Check sheet for the modelled part. Datum: model origin and axes. Units: mm. A direction names the side the tool comes from. Coordinates: 2 decimals unless noted, no trailing zeros. Write each loop counter-clockwise with the first axis right and the second up, starting at its lowest first coordinate (ties: lowest second). Pieces come first, ordered by that corner, then holes. Notation, with made-up numbers: (47, 85.5) - (53, 85.5) arc R20 cw to (53, 112.5) - close; hole circle Ø6 at (26.5, 0.5). An arc over 180 degrees is marked (long way). Use one line per item in the form item = value. Start each with the question number.
1. Draft check along Y on faces 1 (the face through (-1.5, 0.75, 0)), 2 (the face through (0, 1, -1)), 3 (the face through (-0.91, -1.9, -0.08)), 4 (the face through (-1.5, -0.75, 0)). Enter one of: +Y half, -Y half, draft (parallel to the pull), parting line (faces both ways), or undercut.
2. Scan lines: line 1 along X through (y, z) = (1.35, -0.55); line 2 along Y through (x, z) = (6.25, 0.9). Record each from-to range of solid material in increasing order.
3. Go/stop test with a flat-tipped pin: pin 1 Ø1.5 at (x, z) = (4, 1.5) entering from -Y. Record where the tip stops, or that it passes through.
4. Tool access check on faces 5 (the face through (-0.53, 0.05, -0.02)), 6 (the face through (8, 0, 1)). Record the directions out of +Z, -Z, +X, -X, +Y, -Y that give a thin tool (end or side, any length) a straight path to the whole face; none if there is none.
5. Cross-section at A-A on x = 12.5. Record the boundary of the cut face in (y, z), then the cut area to 3 significant figures.
Autodesk Inventor part; units mm, degrees
ref_plane "Work Plane1" through (29, 0, 0) normal (0, -1, 0) x (1, 0, 0)
ref_plane "YZ Plane" through (0, 0, 0) normal (1, 0, 0) x (0, 1, 0)
ref_plane "XZ Plane" through (0, 0, 0) normal (0, 1, 0) x (-1, 0, 0)
sketch "Sketch1" plane through (0, 0, 0) normal (0, 0, 1) x (1, 0, 0)
  line L0 (-0.5, 0) -> (16, 0)
  line L1 (16, 0) -> (16, 1)
  line L2 (16, 1) -> (1, 1)
  line L3 (1, 1) -> (0.7545, 1)
  line L4 (0.7545, 1) -> (0, 1)
  line L5 (0, 1) -> (0, 1.9)
  line L6 (0, 1.9) -> (-2, 1.9)
  line L7 (-2, 1.9) -> (-2, 0.866)
  line L8 (-2, 0.866) -> (-1, 0.866)
  line L9 (-1, 0.866) -> (-0.5, 0)
  line L10 (-5.6, 0) -> (19.6, 0)
  line L11 (0, -0.38) -> (0, 2.28)
  line L12 (1, 1) -> (0, 1) construction
  dimension "d1" = 15
  dimension "d2" = 0.2455
  dimension "d3" = 2
  dimension "d4" = 1
  dimension "d5" = 60
  dimension "d6" = 2
  dimension "d7" = 2
  dimension "d8" = 1.7321
  dimension "d9" = 3.8
  dimension "d26" = 16
revolve "Body" add sketch "Sketch1" angle 360 about axis through (-0.5, 0, 0) along (1, 0, 0)
sketch "Sketch2" plane through (-2, 0, 0) normal (-1, 0, 0) x (0, 0, 1)
  circle A0 centre (0, 0) radius 0.866
  line L0 (0, -2.66) -> (0, 2.66)
  line L1 (-2.66, 0) -> (2.66, 0)
  line L2 (0.866, 0) -> (0.433, -0.75)
  line L3 (0.433, -0.75) -> (-0.433, -0.75)
  line L4 (-0.433, -0.75) -> (-0.866, 0)
  line L5 (-0.866, 0) -> (-0.433, 0.75)
  line L6 (-0.433, 0.75) -> (0.433, 0.75)
  line L7 (0.433, 0.75) -> (0.866, 0)
  point P0 (0, 0)
extrude "Slot" add sketch "Sketch2" against normal up to next contours L7 A0 | A0 L2 | L6 L0 A0 | A0 L0 L3 | L0 L6 A0 | A0 L3 L0 | L4 A0 | A0 L5
fillet "Fillet1" radius 0.2 1 edges at (-2, -1.9, 0)
thread "Thread"
chamfer "Chamfer1" distance 0.2454 distance2 0.2454 1 edges at (16, -1, 0) measured on face at (16, -0.5786, -0.2558)
ref_plane "Work Plane1" through (29, 0, 0) normal (0, -1, 0) x (1, 0, 0)
fillet "Fillet2" radius 0.1 1 edges at (0, -1, 0)
equation "\"d1\" = GEL"
equation "\"d3\" = KOH"
equation "\"d4\" = INTI"
equation "\"d6\" = GD"
equation "\"d7\" = BDM"
equation "\"d8\" = 1.1547 * SW"
equation "\"d9\" = KOD"
equation "\"d26\" = NLG"
equation "\"d30\" = R"
equation "\"d17\" = RR"
equation "\"d13\" = GEL"
equation "\"d15\" = -0.5 * SPD + 0.5 * GD"
equation "\"d16\" = GUL"
equation "\"GD\" = 2"
equation "\"NLG\" = 16"
equation "\"GEL\" = 15"
equation "\"KOD\" = 3.8"
equation "\"KOH\" = 2"
equation "\"INTI\" = 1"
equation "\"GAL\" = 0.61345 * PTC"
equation "\"GUL\" = 0.61345 * PTC"
equation "\"BDM\" = NND"
equation "\"SW\" = 1.5"
equation "\"RR\" = 0.2"
equation "\"SPD\" = NND - 1.2269 * PTC"
equation "\"R\" = 0.1"
equation "\"TOA\" = 30deg"
equation "\"GD1\" = THREADDIA - 1.2269 * PTC"
equation "\"THREADDIA\" = 2"
equation "\"FAWI\" = 45deg"
equation "\"PTC\" = 0.4"
equation "\"NND\" = 2"
equation "\"E0\" = 1.155 * SW"
properties part number "ISO 4762 - M2 x 16" material "Steel"
Final values:
q1.face_1 = undercut
q1.face_2 = draft
q1.face_3 = parting line
q1.face_4 = undercut
q2.line_1 = -2 to 0
q2.line_2 = -0.44 to 0.44
q3.pin_1 = -0.66
q4.face_5 = -X
q4.face_6 = +X
q5.outline = circle Ø2 at (0, 0)
q5.area = 3.14 mm²
